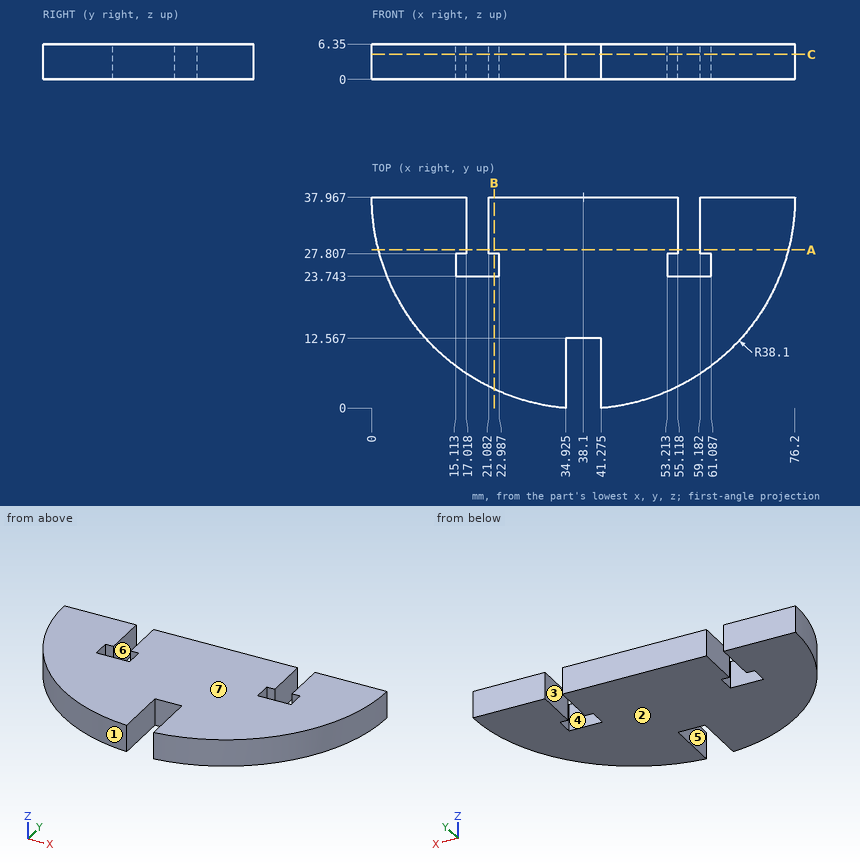
Here's the drawing with two shaded views (mm, measured from the low corner). I have some questions. A direction names the side the tool comes from. Give positions to 0.01 mm unless a question says otherwise; leave off trailing zeros. Loops run counter-clockwise (first coordinate to the right, second up) from the corner with the lowest first, then second, coordinate; pieces in that order, holes last. Notation, with made-up numbers: M 1.5,63.25 L 12.5,63.25 A19 cw 12.5,72.25 Z; hole C -4,29.25 d11. An arc over 180 degrees is marked long. Use one line per item in the form item = value. Start each with the question number.
Q1. If we section it at B-B (x = 22): Write out the boundary of the cut face in (y, z).
Q2. Will these pins go through, and if not, where does the flat tip stop? pin 1 Ø3 at (x, z) = (19.5, 2) entering from +Y; pin 2 Ø1.9 at (y, z) = (8, 2.5) entering from +X; pin 3 Ø1.5 at (y, z) = (24.5, 3) entering from -X (1 decimal).
Q3. I need wall thicknesses on line 1 along X through (y, z) = (32, 2.25); line 2 along X through (y, z) = (25, 3.25) (1 decimal); line 3 along X through (y, z) = (9.5, 2.5) (1 decimal). Which ranges of each line are inside material? Lowest first, please.
Q4. Thinking about a two-plate mould opening in X: for the marked faces 1, 2 and 3, which applies, +X half, -X half, draft (parallel to the pull), parting line (faces both ways), or undercut?
Q5. Which directions (+Z, -Z, +X, -X, +Y, -Y) give clear straight access to the entire face, cutting with the end or side of a thin tool? Please do the marked faces 4, 5, 6 and 7.
Q6. If we section it at A-A (y = 28.5): State how many separate pieces and enclosed holes the cut face has, then the cut area to 3 significant figures.
Q7. If we section it at C-C (z = 4.5): Write out the boundary of the cut face in (x, y) (1 decimal), then the cut area to 3 significant figures.
Taken from the geometry:
q1.outline = M 3.44,0 L 23.74,0 L 23.74,6.35 L 3.44,6.35 Z; M 27.81,0 L 37.97,0 L 37.97,6.35 L 27.81,6.35 Z
q2.pin_1 = 23.74
q2.pin_2 = 62.79
q2.pin_3 = 2.2
q3.line_1 = 0.47 to 17.02, 21.08 to 55.12, 59.18 to 75.73
q3.line_2 = 2.3 to 15.1, 23 to 53.2, 61.1 to 73.9
q3.line_3 = 12.8 to 34.9, 41.3 to 63.4
q4.face_1 = -X half
q4.face_2 = draft
q4.face_3 = undercut
q5.face_4 = +Z, -Z
q5.face_5 = +Z, -Z, -Y
q5.face_6 = +Z, -Z, +Y
q5.face_7 = +Z, +X, -X, +Y, -Y
q6.separate_pieces = 3
q6.enclosed_holes = 0
q6.area = 417 mm^2
q7.outline = M 0,38 A38.1 ccw 34.9,0 L 34.9,12.6 L 41.3,12.6 L 41.3,0 A38.1 ccw 76.2,38 L 59.2,38 L 59.2,27.8 L 61.1,27.8 L 61.1,23.7 L 53.2,23.7 L 53.2,27.8 L 55.1,27.8 L 55.1,38 L 21.1,38 L 21.1,27.8 L 23,27.8 L 23,23.7 L 15.1,23.7 L 15.1,27.8 L 17,27.8 L 17,38 Z
q7.area = 2,050 mm^2
